from build123d import *

# Parameters (mm, degrees)
F0_W     = 25.4
F0_H     = 63.5
F1_DEPTH = 19.05


with BuildPart() as f1:
    # F0 (on Front) → F1 (new body)
    with BuildSketch(Plane.XZ):
        Polygon((-53.701798, 123.424824), (-72.751798, 123.424824), (-72.751798, -130.575176), (-34.651798, -130.575176), (43.184318, -130.575176), (43.184318, 123.424824), (20.14126, 123.424824), (-5.25874, 123.424824), (-34.651798, 123.424824), align=None)
        with Locations((7.44126, 155.174824)):
            Rectangle(F0_W, F0_H)
    extrude(amount=F1_DEPTH)


solid = f1.part
Design review of the part built by this model. Coordinates are the model's own, in mm. A direction names the side the tool comes from. Coordinates: 2 decimals unless noted, no trailing zeros. Loops run counter-clockwise (first coordinate to the right, second up) from the corner with the lowest first, then second, coordinate; pieces in that order, holes last. Notation, with made-up numbers: M -25,81.5 L -10,81.5 A20 ccw -10,103.5 Z; hole C 67.5,-32.5 d10. An arc over 180 degrees is marked long. Answer as CSV lines item,"result".
Item 1: For probe 1 along Z at (x, y) = (26, -9.5); probe 2 along X at (y, z) = (-14.25, 132), list the stretches that pass through material, from the lowest coordinate up.
Answer list:
probe 1,"-130.58 to 123.42"
probe 2,"-5.26 to 20.14"
Item 2: Add section C-C on x = -28. State the section outline as (y, z) points, plus the area to 3 significant figures.
Answer list:
outline,"M -19.05,-130.58 L 0,-130.58 L 0,123.42 L -19.05,123.42 Z"
area,"4,840 mm²"
Item 3: Machinability: for faces 1 (the face through (20.141, -9, 155)), 2 (the face through (-39, -9, 123.425)), 3 (the face through (-72.752, -9, -2)), which of the approach directions +Z, -Z, +X, -X, +Y, -Y give a long, thin tool a straight path to every point of the face, cutting with its end or side? Answer none if there is none.
Answer list:
face 1,"+Z, +X, +Y, -Y"
face 2,"+Z, -X, +Y, -Y"
face 3,"+Z, -Z, -X, +Y, -Y"
Item 4: Add section A-A on y = -13.75. State the section outline as (x, z) points.
Answer list:
outline,"M -72.75,-130.58 L 43.18,-130.58 L 43.18,123.42 L 20.14,123.42 L 20.14,186.92 L -5.26,186.92 L -5.26,123.42 L -72.75,123.42 Z"
Item 5: Add section B-B on z = 146. State the section outline as (x, y) points.
Answer list:
outline,"M -5.26,-19.05 L 20.14,-19.05 L 20.14,0 L -5.26,0 Z"
Item 6: For P1, Ø5.5, axis at x = -46, y = -10, coming from the +Z side; P2, Ø9.5, axis at y = -9, z = 166.5, coming from the -X side; P3, Ø9.5, axis at y = -9.5, z = 166, coming from the +X side, all flat-tipped, find the tip position at first contact; note any pin that passes through.
Answer list:
P1,"z = 123.42"
P2,"x = -5.26"
P3,"x = 20.14"
